Design review of the part built by this model. Coordinates are the model's own, in mm. A direction names the side the tool comes from. Coordinates: 2 decimals unless noted, no trailing zeros. Order: outer loops, then holes, each group sorted by start corner. A loop starts at its lowest first (then second) coordinate and runs counter-clockwise, first axis right, second up. Notation, with made-up numbers: (42, -37) -> (64, -37) arc R29 cw to (64, -4) -> close; hole circle Ø8 at (17, 17.25). An arc over 180 degrees is marked (long way). Write item = value, one per line.
Autodesk Fusion 360 part; units mm, degrees
sketch "cover base" plane through (0, 0, 0) normal (0, 1, 0) x (1, 0, 0)
  line L0 (17.5, -55) -> (-17.5, -55)
  line L1 (-17.5, -55) -> (-17.5, 55)
  line L2 (-17.5, 55) -> (17.5, 55)
  line L3 (17.5, 55) -> (17.5, -55)
  line L4 (17.5, -55) -> (-17.5, 55) construction
  line L5 (-17.5, -55) -> (17.5, 55) construction
  dimension "d1" = 35
  dimension "d2" = 110
extrude "Extrude1" add sketch "cover base" along normal blind 5
sketch "Screw holder" plane through (0, 0, 0) normal (0, -1, 0) x (1, 0, 0)
  line L0 (-17.5, -55) -> (17.5, -55)
  line L1 (17.5, -55) -> (17.5, 55)
  line L2 (17.5, 55) -> (-17.5, 55)
  line L3 (-17.5, 55) -> (-17.5, -55)
  line L4 (7.5, 55) -> (17.5, 55)
  line L5 (17.5, 55) -> (17.5, 65)
  line L6 (17.5, 65) -> (7.5, 65)
  line L7 (7.5, 65) -> (7.5, 55)
  circle A0 centre (12.5, 60) radius 4
  circle A1 centre (12.5, 60) radius 2
  dimension "d5" = 10
  dimension "d6" = 10
  dimension "d9" = 8
  dimension "d10" = 4
extrude "Extrude2" add sketch "Screw holder" against normal blind 5 contours L2 L4 L5 L6 L7 | A0 | A1
extrude "Extrude3" cut sketch "Screw holder" against normal up to surface (5 mm away) contours A1
extrude "Extrude4" cut sketch "Screw holder" against normal blind 3 contours A0
mirror "Mirror1" about plane through (0, 0, 0) normal (0, 0, 1) of "Extrude2", "Extrude3", "Extrude4"
sketch "Slit" plane through (0, 5, 0) normal (0, 1, 0) x (-1, 0, 0)
  circle A0 centre (-12.5, -60) radius 2
  circle A1 centre (-12.5, 60) radius 2
  line L0 (-7.5, -55) -> (17.5, -55)
  line L1 (17.5, -55) -> (17.5, 55)
  line L2 (17.5, 55) -> (-7.5, 55)
  line L3 (-7.5, 55) -> (-7.5, 65)
  line L4 (-7.5, 65) -> (-17.5, 65)
  line L5 (-17.5, 65) -> (-17.5, -65)
  line L6 (-17.5, -65) -> (-7.5, -65)
  line L7 (-7.5, -65) -> (-7.5, -55)
  line L8 (-17.5, 55) -> (11.5, 55) construction
  line L9 (17.5, 45) -> (9.5, 45)
  line L10 (9.5, 45) -> (9.5, -45)
  line L11 (9.5, -45) -> (17.5, -45)
  line L12 (17.5, -45) -> (17.5, 45)
  line L13 (11.5, 55) -> (11.5, 45) construction
  line L14 (12.5, 45) -> (11.5, 45)
  line L15 (11.5, 45) -> (11.5, -45)
  line L16 (11.5, -45) -> (12.5, -45)
  line L17 (12.5, -45) -> (12.5, 45)
  dimension "d16" = 29
  dimension "d23" = 8
  dimension "d35" = 90
  dimension "d36" = 90
  dimension "d37" = 1
extrude "Extrude5" add sketch "Slit" along normal blind 3 contours L1 L9 L11 L12 L17 | L9 L11 L14 L15 L16 L17 | L9 L10 L11 L15
extrude "Extrude8" cut sketch "Slit" along normal blind 3 contours L9 L11 L14 L15 L16 L17
fillet "Fillet1" radius 1 1 edges at (-17.5, 0, 0)
fillet "Fillet2" radius 2 2 edges at (7.5, 2.5, -55) (7.5, 2.5, 55)
fillet "Fillet3" radius 1 1 edges at (-9.5, 5, 0)
sketch "Sketch5" plane through (0, 0, 0) normal (0, -1, 0) x (1, 0, 0)
  line L0 (-16.5, 55) -> (-16.5, -55)
  line L1 (-16.5, -55) -> (5.5, -55)
  arc A0 (7.5, -57) -> (5.5, -55) centre (5.5, -57) ccw
  line L2 (7.5, -57) -> (7.5, -65)
  line L3 (7.5, -65) -> (17.5, -65)
  line L4 (17.5, -65) -> (17.5, 65)
  line L5 (17.5, 65) -> (7.5, 65)
  line L6 (7.5, 65) -> (7.5, 57)
  arc A1 (5.5, 55) -> (7.5, 57) centre (5.5, 57) ccw
  line L7 (5.5, 55) -> (-16.5, 55)
  circle A2 centre (12.5, -60) radius 4
  circle A3 centre (12.5, 60) radius 4
  line L8 (12.5, -60) -> (12.5, -45) construction
  circle A4 centre (12.5, -45) radius 3
  dimension "d29" = 15
  dimension "d30" = 6
extrude "Extrude7" cut sketch "Sketch5" against normal up to surface (5 mm away) contours A4
(1) We need section A-A (x = 12.5). Write out the cut boundary in (y, z), and give its area (3 significant figures).
Report:
outline = (0, -65) -> (5, -65) -> (5, -62) -> (3, -62) -> (3, -64) -> (0, -64) -> close; (0, -56) -> (3, -56) -> (3, -58) -> (5, -58) -> (5, -48) -> (0, -48) -> close; (0, -42) -> (5, -42) -> (5, 58) -> (3, 58) -> (3, 56) -> (0, 56) -> close; (0, 64) -> (3, 64) -> (3, 62) -> (5, 62) -> (5, 65) -> (0, 65) -> close
area = 556 mm²
(2) The part is to be moulded in two halves that separate along X. For faces 4 (the flat face through (13, 2, 65)), 5 (the flat face through (17.5, 2, -1)), 6 (the cylindrical face through (12.24, 3.986, -58.017)), say which applies: released by +X, released by -X, zero draft, split by the parting line, or undercut.
Report:
face_4 = zero draft
face_5 = released by +X
face_6 = undercut
(3) For L1, parallel to Z at x = 12.5, y = 0.95; L2, parallel to Z at x = 12.5, y = 3.5; L3, parallel to X at y = 7.25, z = -1.5, list the stretches that pass through material, from the lowest coordinate up.
Report:
L1 = -65 to -64, -56 to -48, -42 to 56, 64 to 65
L2 = -65 to -62, -58 to -48, -42 to 58, 62 to 65
L3 = -17.5 to -12.5, -11.5 to -9.5
(4) Insertion check: pin 1 (2.5 mm diameter, centred on x = -10.5, y = 6, fed in from -Z); pin 2 (1.5 mm diameter, centred on y = 3.5, z = -61, fed in from -X); pin 3 (2 mm diameter, centred on y = 7.5, z = -14.5, fed in from +X). Each pin has a flat end and moves straight along its axis. Give the tip position at first contact, or say it passes through.
Report:
pin_1 = -55
pin_2 = 7.5
pin_3 = -9.5
(5) For faces 1 (the flat face through (7.5, 2, -61)), 2 (the flat face through (-15, 6, -45)), 3 (the flat face through (-10, 6, 45)), list the 3-axis set-ups (+Z, -Z, +X, -X, +Y, -Y) from which the entire face can be reached by the end or side of a thin tool; tool diameter is ignored.
Report:
face_1 = -Z, -X, +Y, -Y
face_2 = -Z, +X, -X, +Y
face_3 = +Z, +X, -X, +Y
(6) We need section D-D (z = 49). Write out the cut boundary in (x, y).
Report:
outline = (-17.5, 1) arc R1 ccw to (-16.5, 0) -> (17.5, 0) -> (17.5, 5) -> (-17.5, 5) -> close
(7) We need section C-C (z = 0). Write out the cut boundary in (x, y).
Report:
outline = (-17.5, 1) arc R1 ccw to (-16.5, 0) -> (17.5, 0) -> (17.5, 5) -> (-8.5, 5) arc R1 cw to (-9.5, 6) -> (-9.5, 8) -> (-11.5, 8) -> (-11.5, 5) -> (-12.5, 5) -> (-12.5, 8) -> (-17.5, 8) -> close
(8) We need section B-B (z = -60). Write out the cut boundary in (x, y), and give its area (3 significant figures).
Report:
outline = (7.5, 0) -> (8.5, 0) -> (8.5, 3) -> (10.5, 3) -> (10.5, 5) -> (7.5, 5) -> close; (14.5, 3) -> (16.5, 3) -> (16.5, 0) -> (17.5, 0) -> (17.5, 5) -> (14.5, 5) -> close
area = 18.0 mm²
